from build123d import *

# Parameters (mm, degrees)
BOSS_EXTRUDE1_DEPTH = 18
SKETCH3_R           = 1.45
CUT_EXTRUDE1_DEPTH  = 56.244999774
SKETCH5_W           = 22.958144304
SKETCH5_H           = 5
BOSS_EXTRUDE2_DEPTH = 5
SKETCH6_R           = 8.025
CUT_EXTRUDE2_DEPTH  = 55.479353888
SKETCH7_R           = 9
SKETCH7_R_2         = 7
BOSS_EXTRUDE3_DEPTH = 1
FILLET1_R           = 5
FILLET2_R           = 10


with BuildPart() as part:
    # Sketch1 → Boss-Extrude1 (new body)
    with BuildSketch(Plane.XY):
        with BuildLine():
            Line((15.267285286, 1), (28.676455767, 1))
            Line((28.676455767, 1), (28.676455767, 4))
            Line((28.676455767, 4), (18.676455767, 4))
            ThreePointArc((18.676455767, 4), (5.072789326, 18.414038353), (-13.99321264, 13))
            Line((-13.99321264, 13), (-50, 13))
            Line((-50, 13), (-50, 8))
            Line((-50, 8), (-13.041855696, 8))
            ThreePointArc((-13.041855696, 8), (3.67261953, 14.852672008), (15.267285286, 1))
        make_face()
    extrude(amount=BOSS_EXTRUDE1_DEPTH)

    # Sketch3 → Cut-Extrude1 (cut, through all)
    with BuildSketch(Plane(origin=(0, 4, 0), x_dir=(1, 0, 0), z_dir=(0, 1, 0))):
        with Locations(Location((23.676455767, -4, 0), (0, 0, 270))):
            Circle(SKETCH3_R)
        with Locations(Location((23.676455767, -14, 0), (0, 0, 270))):
            Circle(SKETCH3_R)
    extrude(amount=-CUT_EXTRUDE1_DEPTH, mode=Mode.SUBTRACT)

    # Sketch5 → Boss-Extrude2 (add)
    with BuildSketch(Plane.XZ.offset(-8)):
        with Locations((-38.520927848, -2.5)):
            Rectangle(SKETCH5_W, SKETCH5_H)
    extrude(amount=-BOSS_EXTRUDE2_DEPTH)

    # Sketch6 → Cut-Extrude2 (cut, through all)
    with BuildSketch(Plane(origin=(0, 13, 0), x_dir=(1, 0, 0), z_dir=(0, 1, 0))):
        with Locations(Location((-37, -6, 0), (0, 0, 180))):
            Circle(SKETCH6_R)
    extrude(amount=-CUT_EXTRUDE2_DEPTH, mode=Mode.SUBTRACT)

    # Sketch7 → Boss-Extrude3 (add)
    with BuildSketch(Plane.XZ.offset(-8)):
        with Locations(Location((-37, 6, 0), (0, 0, 180))):
            Circle(SKETCH7_R)
        with Locations((-37, 6)):
            Circle(SKETCH7_R_2, mode=Mode.SUBTRACT)
    extrude(amount=BOSS_EXTRUDE3_DEPTH)

    # Fillet1
    fillet1_edges = [part.edges().sort_by_distance(p)[0] for p in [
        (-50, 10.5, 18),
        (-50, 10.5, -5),
    ]]
    fillet(fillet1_edges, radius=FILLET1_R)

    # Fillet2
    # the kernel refuses this fillet: 10 mm, written as the material it takes off along each edge
    with BuildSketch(Plane(origin=(-27.041855696, -13.650635095, -5), x_dir=(0, 0, 1), z_dir=(0, 1, 0))) as fillet2_piece_1:
        with BuildLine():
            CenterArc((10, -8.660254038), FILLET2_R, 120, 60)
            Line((0, -8.660254038), (-0.2, -8.660254038))
            Line((-0.2, -8.660254038), (-0.2, 0))
            Line((-0.2, 0), (0, 0.2))
            ThreePointArc((0, 0.2), (2.5, 0.2), (4.9, 0.173205081))
            Line((4.9, 0.173205081), (5, 0))
        make_face()
    extrude(amount=48.301270189, mode=Mode.SUBTRACT)


solid = part.part
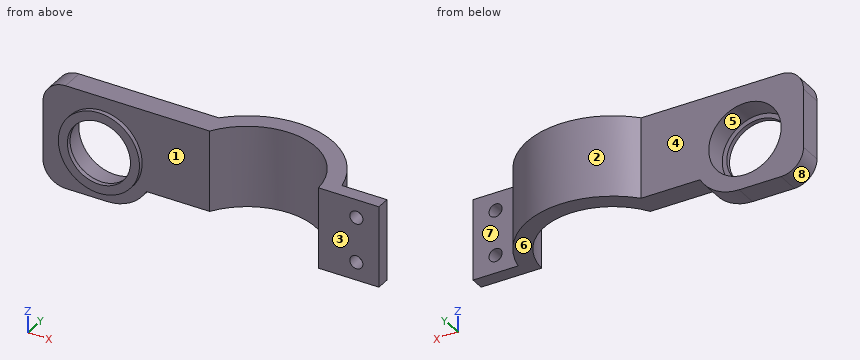
Part model, mm, in its own coordinate system. Face numbers are marked on the shaded views. A direction names the side the tool comes from. Give positions to 0.01 mm unless a question says otherwise; leave off trailing zeros. Order: outer loops, then holes, each group sorted by start corner. A loop starts at its lowest first (then second) coordinate and runs counter-clockwise, first axis right, second up. Notation, with made-up numbers: (-31.5, 35.25) - (2.5, 35.25) arc R11 cw to (2.5, 46.25) - close; hole circle Ø8 at (-20.5, 15.25). An arc over 180 degrees is marked (long way). Use a Markdown table: item, result.
1) Flat gauge pins, fed straight in: P1, Ø1.5, axis at x = -29, y = 6.5, coming from the +Z side; P2, Ø8, axis at y = 10, z = 5.5, coming from the +X side; P3, Ø6, axis at y = 7.5, z = 0.5, coming from the +X side. Where does each tip first touch, or does it go through?
Checked values:
| item | result |
|---|---|
| P1 | z = 11.06 |
| P2 | x = 18.13 |
| P3 | x = 18.56 |
2) Saw through at D-D on z = 4. List the corners of the cut face in (x, y), plus the area to 3 significant figures.
Checked values:
| item | result |
|---|---|
| outline | (-50, 8) - (-45.77, 8) - (-45.77, 7) - (-43.71, 7) - (-43.71, 8) - (-44.77, 8) - (-44.77, 13) - (-50, 13) - close; (-30.29, 7) - (-28.23, 7) - (-28.23, 8) - (-13.04, 8) arc R15.3 cw to (15.27, 1) - (22.23, 1) - (22.23, 4) - (18.68, 4) arc R19.1 ccw to (-13.99, 13) - (-29.23, 13) - (-29.23, 8) - (-30.29, 8) - close; (25.13, 1) - (28.68, 1) - (28.68, 4) - (25.13, 4) - close |
| area | 288 mm² |
3) Two-plate mould, pull along X, no slides. Class the marked faces 1, 2 and 3: +X half, -X half, draft (parallel to the pull), parting line (faces both ways), or undercut.
Checked values:
| item | result |
|---|---|
| face 1 | undercut |
| face 2 | parting line |
| face 3 | draft |
4) Saw through at C-C on x = -32.5. List the corners of the cut face in (y, z).
Checked values:
| item | result |
|---|---|
| outline | (7, -1.79) - (8, -1.79) - (8, -4.47) - (13, -4.47) - (13, -0.64) - (8, -0.64) - (8, 0.64) - (7, 0.64) - close; (7, 11.36) - (8, 11.36) - (8, 12.64) - (13, 12.64) - (13, 18) - (8, 18) - (8, 13.79) - (7, 13.79) - close |
5) Saw through at B-B on z = 9.5. List the corners of the cut face in (x, y).
Checked values:
| item | result |
|---|---|
| outline | (-50, 8) - (-45.29, 8) - (-45.29, 7) - (-43.06, 7) - (-43.06, 8) - (-44.22, 8) - (-44.22, 13) - (-50, 13) - close; (-30.94, 7) - (-28.71, 7) - (-28.71, 8) - (-13.04, 8) arc R15.3 cw to (15.27, 1) - (28.68, 1) - (28.68, 4) - (18.68, 4) arc R19.1 ccw to (-13.99, 13) - (-29.78, 13) - (-29.78, 8) - (-30.94, 8) - close |
6) 3-axis set-ups, long thin cutter, end or side, ignore diameter. For the marked faces 4, 5, 6, 7 and 8: which of +Z, -Z, +X, -X, +Y, -Y reach the whole face in a straight line?
Checked values:
| item | result |
|---|---|
| face 4 | +Z, -Z, -X, +Y |
| face 5 | +Y |
| face 6 | -Z, +X, +Y, -Y |
| face 7 | +Z, -Z, +X, +Y |
| face 8 | -Z, -X, +Y, -Y |
7) Saw through at A-A on y = 11.25. List the corners of the cut face in (x, z) (3 decimals), plus the area to 3 significant figures.
Checked values:
| item | result |
|---|---|
| outline | (-50, 0) arc R5 ccw to (-45, -5) - (-35.702, -5) arc R10 ccw to (-27.042, 0) - (-10.37, 0) - (-10.37, 18) - (-45, 18) arc R5 ccw to (-50, 13) - close; (10.37, 0) - (15.435, 0) - (15.435, 18) - (10.37, 18) - close; hole circle Ø16.05 at (-37, 6) |
| area | 694 mm² |
8) Probe L1, parallel to Z at x = -37, y = 9.1 (3 decimals); L2, parallel to Z at x = -37, y = 7.4; L3, parallel to Y at x = -42, z = -1. List the from-to ranges inside material, lowest first. Write a range as from..to.
Checked values:
| item | result |
|---|---|
| L1 | -5..-2.025, 14.025..18 |
| L2 | -3..-1, 13..15 |
| L3 | 7..13 |
